Verification items for this drawing (mm, ordinates from the low corner). Give positions to 0.01 mm unless a question says otherwise; leave off trailing zeros. Write each loop counter-clockwise with the first axis right and the second up, starting at its lowest first coordinate (ties: lowest second). Pieces come first, ordered by that corner, then holes. Notation, with made-up numbers: (-7.75, 65.5) -> (27.25, 65.5) arc R22 ccw to (27.25, 98.5) -> close; hole circle Ø1 at (63.5, -39). An arc over 180 degrees is marked (long way). One line per item, written item: value.
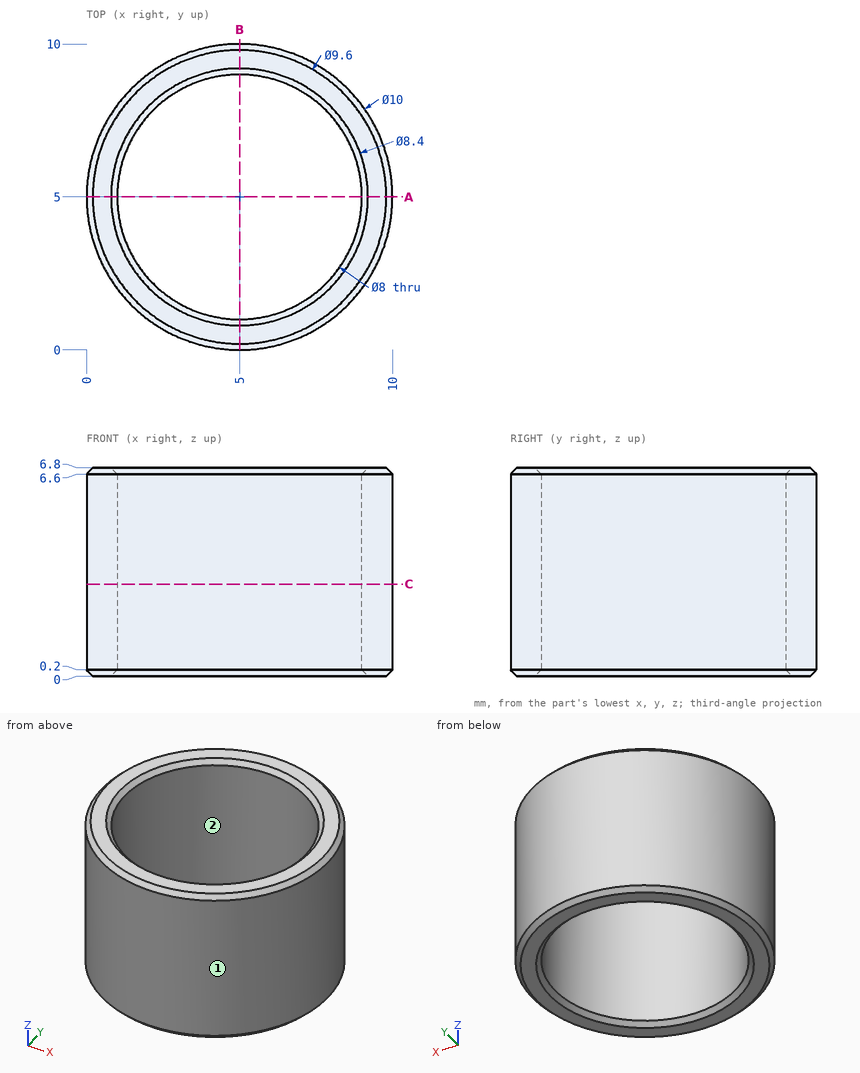
1) Mould release check, pull along X, two halves, no side actions. Record for the marked faces 1 and 2: released by +X, released by -X, zero draft, split by the parting line, or undercut.
Verdict:
face 1: split by the parting line
face 2: undercut
2) Sectioned sample at C-C on z = 3. Record the cut outline in (x, y).
Verdict:
outline: circle Ø10 at (5, 5); hole circle Ø8 at (5, 5)
3) Sectioned sample at A-A on y = 5. Record the cut outline in (x, z).
Verdict:
outline: (0, 0.2) -> (0.2, 0) -> (0.8, 0) -> (1, 0.2) -> (1, 6.6) -> (0.8, 6.8) -> (0.2, 6.8) -> (0, 6.6) -> close; (9, 0.2) -> (9.2, 0) -> (9.8, 0) -> (10, 0.2) -> (10, 6.6) -> (9.8, 6.8) -> (9.2, 6.8) -> (9, 6.6) -> close
4) Depth check by flat-ended pin: pin 1 Ø4 at (y, z) = (1.5, 2) entering from +X; pin 2 Ø1 at (y, z) = (3.5, 6) entering from +X. Enter the tip coordinate at first touch or a pass-through.
Verdict:
pin 1: x = 9.77
pin 2: x = 9.9
5) Scan lines: probe 1 along Y at (x, z) = (5, 4.75); probe 2 along X at (y, z) = (7.5, 2.5); probe 3 along X at (y, z) = (3.5, 1.75). Record each from-to range of solid material in increasing order.
Verdict:
probe 1: 0 to 1, 9 to 10
probe 2: 0.67 to 1.88, 8.12 to 9.33
probe 3: 0.23 to 1.29, 8.71 to 9.77
